The listing builds one solid part. Answer for the finished solid, in the listing's coordinates (mm). Face numbers are marked on the shaded views. A direction names the side the tool comes from. Round coordinates to 2 decimals unless told otherwise and drop trailing zeros. Write each loop counter-clockwise with the first axis right and the second up, starting at its lowest first coordinate (ties: lowest second). Pieces come first, ordered by that corner, then holes. Notation, with made-up numbers: (82.25, 54) - (132.25, 54) arc R15 ccw to (132.25, 80) - close; hole circle Ø6 at (56, 22). An arc over 180 degrees is marked (long way). Use a Markdown table: item, result. Add a question column.
1) Find the intervals of material crossed by probe 1 along Z at (x, y) = (0, 5); probe 2 along X at (y, z) = (-3.5, -5.75); probe 3 along Z at (x, y) = (-3.75, 6.75), in increasing order. Write a range as from..to.
2) A cutting plane is placed at D-D (z = -8.25). Give the vertices of the cut face in (x, y), then the cut area to 3 significant figures.
3) A cutting plane is placed at A-A (z = 0). Give the vertices of the cut face in (x, y), then the cut area to 3 significant figures.
4) Each of these flat-tipped pins is pushed along its axis until it touches: P1, Ø8, axis at y = 3.5, z = -7, coming from the -X side; P2, Ø12, axis at x = 2, z = -1.5, coming from the -Y side; P3, Ø1, axis at x = 2.5, z = -11.5, coming from the -Y side; P4, Ø10, axis at x = 4, z = -9.5, coming from the -Y side. Where does it stop, or does it pass through?
5) Determine the mould class of the marked faces 4, 5 and 6 for opening direction X: +X half, -X half, draft (parallel to the pull), parting line (faces both ways), or undercut.
6) A cutting plane is placed at B-B (x = 0). Give the vertices of the cut face in (y, z).
7) A cutting plane is placed at C-C (y = -2.75). Give the vertices of the cut face in (x, z), then the cut area to 3 significant figures.
8) A tool of negligible diameter and unlimited length cuts with its end or side. For the marked faces 1, 2 and 3, from which of +Z, -Z, +X, -X, +Y, -Y can it reach the whole face along a straight path? Write none if from no direction.
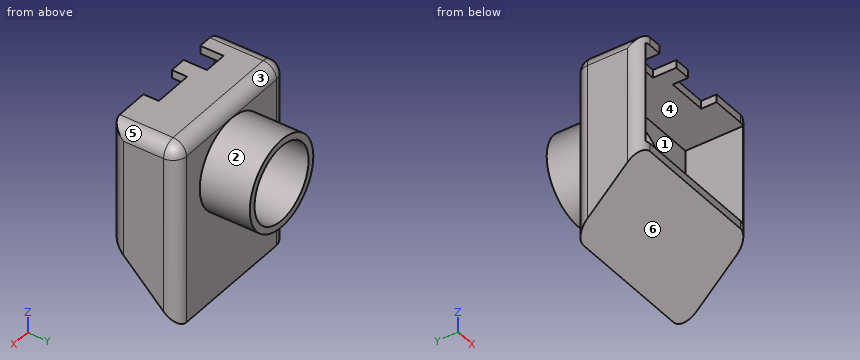
```python
from build123d import *

# Parameters (mm, degrees)
F0_W          = 23
F0_H          = 17.5
F1_DEPTH      = 10
F2_T          = -1.2
F3_R          = 5.7
F4_DEPTH      = 3
F3_R_2        = 6.7
F5_DEPTH      = 7.5
F6_W          = 6
F6_H          = 2.3
F6_W_2        = 3.5
F6_H_2        = 3.5
F7_DEPTH      = 4
F8_DEPTH      = 10
F10_DEPTH     = 30
F11_T1_DEPTH  = 19
F11_T3_DEPTH  = 30.5
F11_T5_DEPTH  = 13
F11_T7_DEPTH  = 27.5
F11_S11_W     = 2
F11_S11_H     = 2
F11_T12_DEPTH = 2
F11_S17_W     = 2
F11_S17_H     = 2
F11_T18_DEPTH = 2


# Not quite as in the source:
# - a fillet or chamfer that OpenCascade refuses, or shapes differently, is made with other operations: its cross-section is extruded or revolved along the edge and cut away or added


with BuildPart() as f1:
    # F0 (on Front) → F1 (new body)
    with BuildSketch(Plane.XZ):
        Rectangle(F0_W, F0_H)
    extrude(amount=F1_DEPTH)

    # F2
    f2_openings = [f1.faces().sort_by_distance(p)[0] for p in [
        (0, -10, 0),
    ]]
    offset(amount=F2_T, openings=f2_openings)

    # F3 (on face) → F4 (cut)
    with BuildSketch(Plane(origin=(0, 0, 0), x_dir=(-1, 0, 0), z_dir=(0, 1, 0))):
        Circle(F3_R)
    extrude(amount=-F4_DEPTH, mode=Mode.SUBTRACT)

    # F3 (on face) → F5 (join)
    with BuildSketch(Plane(origin=(0, 0, 0), x_dir=(-1, 0, 0), z_dir=(0, 1, 0))):
        Circle(F3_R_2)
        Circle(F3_R, mode=Mode.SUBTRACT)
    extrude(amount=F5_DEPTH)

    # F6 (on face) → F7 (cut)
    with BuildSketch(Plane.XY.offset(8.75)):
        with Locations((1.5, -8.85)):
            Rectangle(F6_W, F6_H)
        with Locations((-5.75, -8.25)):
            Rectangle(F6_W_2, F6_H_2)
    extrude(amount=-F7_DEPTH, mode=Mode.SUBTRACT)

    # F8 (add): a face of the model
    f8_faces = [f1.faces().sort_by_distance(p)[0] for p in [
        (0, -5, -8.75),
    ]]
    extrude(f8_faces, amount=F8_DEPTH)

    # F9 (on face) → F10 (cut)
    with BuildSketch(Plane.YZ.offset(11.5)):
        Polygon((-10, -18.75), (0, -18.75), (-10, -8.75), align=None)
    extrude(amount=-F10_DEPTH, mode=Mode.SUBTRACT)

    # F11: fillet of radius 2 on 7 edges, made by hand

    # F11_s2 → F11_t1 (cut)
    with BuildSketch(Plane.YZ.offset(-9.5)):
        with BuildLine():
            ThreePointArc((0, 6.75), (-0.5857864376, 8.1642135624), (-2, 8.75))
            Line((-2, 8.75), (0, 8.75))
            Line((0, 8.75), (0, 6.75))
        make_face()
    extrude(amount=F11_T1_DEPTH, mode=Mode.SUBTRACT)

    # F11_s4 → F11_t3 (cut)
    with BuildSketch(Plane.XY.offset(-23.75)):
        with BuildLine():
            ThreePointArc((-11.5, -2), (-10.9142135624, -0.5857864376), (-9.5, 0))
            Line((-9.5, 0), (-11.5, 0))
            Line((-11.5, 0), (-11.5, -2))
        make_face()
        with BuildLine():
            ThreePointArc((9.5, 0), (10.9142135624, -0.5857864376), (11.5, -2))
            Line((11.5, -2), (11.5, 0))
            Line((11.5, 0), (9.5, 0))
        make_face()
    extrude(amount=F11_T3_DEPTH, mode=Mode.SUBTRACT)

    # F11_s6 → F11_t5 (cut)
    with BuildSketch(Plane.XZ.offset(2)):
        with BuildLine():
            ThreePointArc((9.5, 8.75), (10.9142135624, 8.1642135624), (11.5, 6.75))
            Line((11.5, 6.75), (11.5, 8.75))
            Line((11.5, 8.75), (9.5, 8.75))
        make_face()
        with BuildLine():
            ThreePointArc((-11.5, 6.75), (-10.9142135624, 8.1642135624), (-9.5, 8.75))
            Line((-9.5, 8.75), (-11.5, 8.75))
            Line((-11.5, 8.75), (-11.5, 6.75))
        make_face()
    extrude(amount=F11_T5_DEPTH, mode=Mode.SUBTRACT)

    # F11_s8 → F11_t7 (cut)
    with BuildSketch(Plane.XY.offset(-13.75)):
        with BuildLine():
            ThreePointArc((9.5, -10), (10.9142135624, -9.4142135624), (11.5, -8))
            Line((11.5, -8), (11.5, -10))
            Line((11.5, -10), (9.5, -10))
        make_face()
        with BuildLine():
            ThreePointArc((-11.5, -8), (-10.9142135624, -9.4142135624), (-9.5, -10))
            Line((-9.5, -10), (-11.5, -10))
            Line((-11.5, -10), (-11.5, -8))
        make_face()
    extrude(amount=F11_T7_DEPTH, mode=Mode.SUBTRACT)


with BuildPart() as f11_tool10:
    # F11_s11 → F11_t12 (new body)
    with BuildSketch(Plane.XZ.offset(2)):
        with Locations((10.5, 7.75)):
            Rectangle(F11_S11_W, F11_S11_H)
    extrude(amount=-F11_T12_DEPTH)

    # F11_s13 → F11_t14 (revolve, cut)
    with BuildSketch(Plane(origin=(9.5, -2, 6.75), x_dir=(-0.7071067812, 0, -0.7071067812), z_dir=(0.7071067812, 0, -0.7071067812))):
        with BuildLine():
            ThreePointArc((0, -2), (2, 0), (0, 2))
            Line((0, 2), (0, -2))
        make_face()
    revolve(axis=Axis((9.5, -2, 6.75), (0, 1, 0)), mode=Mode.SUBTRACT)


with BuildPart() as f1_1:
    add(f1.part)

    # F11_t9: cut F11_tool10
    add(f11_tool10.part, mode=Mode.SUBTRACT)


with BuildPart() as f11_tool16:
    # F11_s17 → F11_t18 (new body)
    with BuildSketch(Plane.YZ.offset(-9.5)):
        with Locations((-1, 7.75)):
            Rectangle(F11_S17_W, F11_S17_H)
    extrude(amount=-F11_T18_DEPTH)

    # F11_s19 → F11_t20 (revolve, cut)
    with BuildSketch(Plane(origin=(-9.5, -2, 6.75), x_dir=(0, -0.7071067812, -0.7071067812), z_dir=(0, 0.7071067812, -0.7071067812))):
        with BuildLine():
            ThreePointArc((0, -2), (2, 0), (0, 2))
            Line((0, 2), (0, -2))
        make_face()
    revolve(axis=Axis((-9.5, -2, 6.75), (-1, 0, 0)), mode=Mode.SUBTRACT)


with BuildPart() as f1_2:
    add(f1_1.part)

    # F11_t15: cut F11_tool16
    add(f11_tool16.part, mode=Mode.SUBTRACT)


solid = f1_2.part
```
Entries:
| question | item | result |
|---|---|---|
| 1 | probe 1 | z = -6.7..-5.7, 5.7..6.7 |
| 1 | probe 2 | x = -11.5..-10.3, 10.3..11.5 |
| 1 | probe 3 | z = -5.55..-4.29, 4.29..5.55 |
| 2 | outline | (-11.5, -8) arc R2 ccw to (-9.5, -10) - (9.5, -10) arc R2 ccw to (11.5, -8) - (11.5, -2) arc R2 ccw to (9.5, 0) - (-9.5, 0) arc R2 ccw to (-11.5, -2) - close |
| 2 | area | 227 mm² |
| 3 | outline | (-11.5, -8) arc R2 ccw to (-10.3, -9.83) - (-10.3, -1.2) - (-5.7, -1.2) - (-5.7, 7.5) - (-6.7, 7.5) - (-6.7, 0) - (-9.5, 0) arc R2 ccw to (-11.5, -2) - close; (5.7, -1.2) - (10.3, -1.2) - (10.3, -9.83) arc R2 ccw to (11.5, -8) - (11.5, -2) arc R2 ccw to (9.5, 0) - (6.7, 0) - (6.7, 7.5) - (5.7, 7.5) - close |
| 3 | area | 46.7 mm² |
| 4 | P1 | stops at x = -10.82 |
| 4 | P2 | stops at y = -1.2 |
| 4 | P3 | stops at y = -7.75 |
| 4 | P4 | stops at y = -10 |
| 5 | face 4 | undercut |
| 5 | face 5 | +X half |
| 5 | face 6 | draft |
| 6 | outline | (-10, -8.75) - (0, -18.75) - (0, -6.7) - (7.5, -6.7) - (7.5, -5.7) - (-1.2, -5.7) - (-1.2, -7.55) - (-10, -7.55) - close; (-7.7, 7.55) - (-1.2, 7.55) - (-1.2, 5.7) - (7.5, 5.7) - (7.5, 6.7) - (0, 6.7) - (0, 6.75) arc R2 ccw to (-2, 8.75) - (-7.7, 8.75) - close |
| 7 | outline | (-11.5, -16) - (11.5, -16) - (11.5, 6.75) arc R2 ccw to (9.5, 8.75) - (-9.5, 8.75) arc R2 ccw to (-11.5, 6.75) - close; hole (-10.3, -7.55) - (10.3, -7.55) - (10.3, 7.55) - (-10.3, 7.55) - close |
| 7 | area | 256 mm² |
| 8 | face 1 | -Y |
| 8 | face 2 | +Y |
| 8 | face 3 | +Z, +X, -X, +Y |
